Verification items for the finished model (mm, model axes). Face numbers are marked on the shaded views. A direction names the side the tool comes from. Coordinates: 2 decimals unless noted, no trailing zeros. Write each loop counter-clockwise with the first axis right and the second up, starting at its lowest first coordinate (ties: lowest second). Pieces come first, ordered by that corner, then holes. Notation, with made-up numbers: (48.5, -29.75) - (86.5, -29.75) arc R31 ccw to (86.5, -2.75) - close; hole circle Ø10 at (63, 23). An arc over 180 degrees is marked (long way). Use one line per item in the form item = value. Start each with the question number.
(1) Sectioned sample at B-B (x = 46.5). Count the separate pieces of the cut face and the enclosed holes in it, and give its area (3 significant figures).
(2) Material ranges on line 1 (Y direction, x = 51, z = -2.75); line 2 (X direction, y = 10, z = 0.25); line 3 (X direction, y = 15.5, z = -1), recorded low to high. Write a range as [from, to].
(3) Gauge pin test, flat ends, axial feed: pin 1 Ø0.7 at (x, z) = (2, 9.5) entering from +Y; pin 2 Ø4.5 at (y, z) = (12.5, -2.5) entering from -X; pin 3 Ø6 at (x, z) = (40.5, 5) entering from -Y. Record the tip position at first contact, or that the pin passes through.
(4) Tool access check on the marked faces 4, 5 and 6. Record the directions out of +Z, -Z, +X, -X, +Y, -Y that give a thin tool (end or side, any length) a straight path to the whole face; none if there is none.
(5) Mould release check, pull along X, two halves, no side actions. Record for the marked faces 1, 2 and 3: released by +X, released by -X, zero draft, split by the parting line, or undercut.
(6) Sectioned sample at A-A (z = 3.75). Record the cut outline in (x, y), and give its area (3 significant figures).
from build123d import *

# Parameters (mm, degrees)
BOSS_EXTRUDE1_DEPTH  = 10.8
BOSS_EXTRUDE2_DEPTH  = 1
SKETCH3_W            = 2
SKETCH3_H            = 10
BOSS_EXTRUDE3_DEPTH  = 2.3
FILLET1_SIZE         = 2
FILLET1_SIZE_2       = 1
CUT_EXTRUDE1_REACH   = 67.321
SKETCH4_W            = 11.5
SKETCH4_H            = 3
BOSS_EXTRUDE4_DEPTH  = 2.3
CHAMFER1_SIZE        = 1.5
CUT_EXTRUDE2_DEPTH   = 2
BOSS_EXTRUDE6_DEPTH  = 2
FILLET2_R            = 1
BOSS_EXTRUDE36_DEPTH = 1
BOSS_EXTRUDE7_DEPTH  = 1.87
SKETCH11_R           = 2.5
CUT_EXTRUDE3_DEPTH   = 66.681732761


with BuildPart() as part:
    # Sketch1 → Boss-Extrude1 (new body)
    with BuildSketch(Plane.XY):
        with BuildLine():
            ThreePointArc((7.5, 17.5), (2.196699141, 15.303300859), (0, 10))
            Line((0, 10), (0, 0))
            Line((0, 0), (1.5, 0))
            Line((1.5, 0), (1.5, 10))
            ThreePointArc((1.5, 10), (3.257359313, 14.242640687), (7.5, 16))
            Line((7.5, 16), (54.5, 16))
            ThreePointArc((54.5, 16), (58.742640687, 14.242640687), (60.5, 10))
            Line((60.5, 10), (60.5, 0))
            Line((60.5, 0), (62, 0))
            Line((62, 0), (62, 17.5))
            Line((62, 17.5), (7.5, 17.5))
        make_face()
    extrude(amount=BOSS_EXTRUDE1_DEPTH)


with BuildPart() as body_2:
    # Sketch2 → Boss-Extrude2 (new body)
    with BuildSketch(Plane(origin=(0, 0, 0), x_dir=(-1, 0, 0), z_dir=(0, 0, -1))):
        with BuildLine():
            Line((-1.5, 0), (-1.5, 10))
            ThreePointArc((-1.5, 10), (-3.257359313, 14.242640687), (-7.5, 16))
            Line((-7.5, 16), (-54.5, 16))
            ThreePointArc((-54.5, 16), (-58.742640687, 14.242640687), (-60.5, 10))
            Line((-60.5, 10), (-60.5, 0))
            Line((-60.5, 0), (-1.5, 0))
        make_face()
    extrude(amount=-BOSS_EXTRUDE2_DEPTH)

    # Combine1: union part
    add(part.part)

    # Sketch3 → Boss-Extrude3 (add)
    with BuildSketch(Plane.XY.offset(10.8)):
        with Locations((2.5, 5)):
            Rectangle(SKETCH3_W, SKETCH3_H)
        with Locations((59.5, 5)):
            Rectangle(SKETCH3_W, SKETCH3_H)
    extrude(amount=-BOSS_EXTRUDE3_DEPTH)

    # Fillet1
    # a fillet whose section is not a circle: 2, 1 mm, written as the material it takes off along each edge
    with BuildSketch(Plane(origin=(0, 10, 10.8), x_dir=(0, 0, -1), z_dir=(0, -1, 0))) as fillet1_piece_1:
        with BuildLine():
            Bezier((FILLET1_SIZE, 0), (0, 0), (0, FILLET1_SIZE_2), weights=[1, 0.707106781, 1])
            Line((0, FILLET1_SIZE_2), (0, 0))
            Line((0, 0), (FILLET1_SIZE, 0))
        make_face()
    extrude(amount=15, mode=Mode.SUBTRACT)
    with BuildSketch(Plane(origin=(7.5, 10, 10.8), x_dir=(0, 1, 0), z_dir=(1, 0, 0))) as fillet1_piece_2:
        with BuildLine():
            Bezier((7.5, -FILLET1_SIZE), (7.5, 0), (7.5 - FILLET1_SIZE_2, 0), weights=[1, 0.707106781, 1])
            Line((7.5 - FILLET1_SIZE_2, 0), (7.5, 0))
            Line((7.5, 0), (7.5, -FILLET1_SIZE))
        make_face()
    revolve(axis=Axis((7.5, 10, 10.8), (0, 0, 1)), revolution_arc=90, mode=Mode.SUBTRACT)
    with BuildSketch(Plane(origin=(67, 17.5, 10.8), x_dir=(0, 0, -1), z_dir=(-1, 0, 0))) as fillet1_piece_3:
        with BuildLine():
            Bezier((FILLET1_SIZE, 0), (0, 0), (0, FILLET1_SIZE_2), weights=[1, 0.707106781, 1])
            Line((0, FILLET1_SIZE_2), (0, 0))
            Line((0, 0), (FILLET1_SIZE, 0))
        make_face()
    extrude(amount=59.5, mode=Mode.SUBTRACT)

    # Sketch4 → Cut-Extrude1 (cut, up to next)
    with BuildSketch(Plane(origin=(0, 17.5, 0), x_dir=(1, 0, 0), z_dir=(0, 1, 0)), mode=Mode.PRIVATE) as cut_extrude1_sk1:
        with Locations((45.75, -4.55)):
            Rectangle(SKETCH4_W, SKETCH4_H)
    cut_extrude1_tool1 = extrude(cut_extrude1_sk1.sketch, amount=-CUT_EXTRUDE1_REACH, mode=Mode.PRIVATE) & body_2.part
    add(cut_extrude1_tool1.solids().sort_by_distance((45.75, 17.5, 4.55))[0], mode=Mode.SUBTRACT)

    # Sketch5 → Boss-Extrude4 (add)
    with BuildSketch(Plane.XY.offset(10.8)):
        with BuildLine():
            Line((60.5, 10), (59.5, 10))
            ThreePointArc((59.5, 10), (58.035533906, 13.535533906), (54.5, 15))
            Line((54.5, 15), (7.5, 15))
            ThreePointArc((7.5, 15), (3.964466094, 13.535533906), (2.5, 10))
            Line((2.5, 10), (1.5, 10))
            ThreePointArc((1.5, 10), (3.257359313, 14.242640687), (7.5, 16))
            Line((7.5, 16), (54.5, 16))
            ThreePointArc((54.5, 16), (58.742640687, 14.242640687), (60.5, 10))
        make_face()
    extrude(amount=-BOSS_EXTRUDE4_DEPTH)

    # Chamfer1
    chamfer1_edges = [body_2.edges().sort_by_distance(p)[0] for p in [
        (58.035533906, 13.535533906, 10.8),
        (3.964466094, 13.535533906, 10.8),
        (31, 15, 10.8),
    ]]
    chamfer(chamfer1_edges, length=CHAMFER1_SIZE - 0.0001)  # a hair under: the kernel refuses the full size

    # Chamfer3: read off the stored shape, not the designer's step
    # Chamfer3: loft between two sections, ruled curve by curve
    chamfer3_from = [
        Edge.make_three_point_arc((2.4, 10, 9.4), (3.893755416, 13.606244584, 9.4), (7.5, 15.1, 9.4)),
        Edge.make_three_point_arc((54.5, 15.1, 9.4), (58.106244584, 13.606244584, 9.4), (59.6, 10, 9.4)),
        Edge.make_line((7.5, 15.1, 9.4), (54.5, 15.1, 9.4)),
        Edge.make_line((59.6, 10, 9.4), (2.4, 10, 9.4)),
    ]
    chamfer3_to = [
        Edge.make_three_point_arc((1.5, 10, 8.5), (3.257359313, 14.242640687, 8.5), (7.5, 16, 8.5)),
        Edge.make_three_point_arc((54.5, 16, 8.5), (58.742640687, 14.242640687, 8.5), (60.5, 10, 8.5)),
        Edge.make_line((7.5, 16, 8.5), (54.5, 16, 8.5)),
        Edge.make_line((60.5, 10, 8.5), (1.5, 10, 8.5)),
    ]
    chamfer3 = Solid(Shell([*[Face.make_surface_from_curves(chamfer3_from[k], chamfer3_to[k]) for k in range(4)], Face(Wire(chamfer3_from)), Face(Wire(chamfer3_to))]))
    add(chamfer3, mode=Mode.SUBTRACT)

    # Sketch6 → Cut-Extrude2 (cut)
    with BuildSketch(Plane(origin=(0, 0, 0), x_dir=(-1, 0, 0), z_dir=(0, 0, -1))):
        with BuildLine():
            Line((-59.98, 10.15), (-59.98, 16.85))
            Line((-59.98, 16.85), (-59.98, 17.5))
            Line((-59.98, 17.5), (-42.02, 17.5))
            Line((-42.02, 17.5), (-42.02, 16.85))
            Line((-42.02, 16.85), (-42.02, 10.15))
            ThreePointArc((-42.02, 10.15), (-51, 1.17), (-59.98, 10.15))
        make_face()
    extrude(amount=-CUT_EXTRUDE2_DEPTH, mode=Mode.SUBTRACT)

    # Sketch9 → Boss-Extrude6 (add)
    with BuildSketch(Plane(origin=(0, 0, 0), x_dir=(-1, 0, 0), z_dir=(0, 0, -1))):
        with BuildLine():
            Line((-54.5, 0), (-62, 0))
            Line((-62, 0), (-62, 6.85))
            Line((-62, 6.85), (-62, 17.5))
            Line((-62, 17.5), (-59.98, 17.5))
            Line((-59.98, 17.5), (-59.98, 10.15))
            ThreePointArc((-59.98, 10.15), (-51, 1.17), (-42.02, 10.15))
            Line((-42.02, 10.15), (-42.02, 17.5))
            Line((-42.02, 17.5), (-40, 17.5))
            Line((-40, 17.5), (-40, 6.854472052))
            Line((-40, 6.854472052), (-40, 0))
            Line((-40, 0), (-47.292116273, 0))
            Line((-47.292116273, 0), (-54.5, 0))
        make_face()
    extrude(amount=BOSS_EXTRUDE6_DEPTH)

    # Fillet2
    fillet2_edges = [body_2.edges().sort_by_distance(p)[0] for p in [
        (51.5, 17.5, 4.55),
        (45.75, 17.5, 3.05),
        (40, 17.5, 4.55),
        (45.75, 17.5, 6.05),
    ]]
    fillet(fillet2_edges, radius=FILLET2_R)

    # Sketch48 → Boss-Extrude36 (add)
    with BuildSketch(Plane(origin=(0, 0, 2), x_dir=(-1, 0, 0), z_dir=(0, 0, -1))):
        with BuildLine():
            Line((-54.5, 16), (-42.02, 16))
            Line((-42.02, 16), (-42.02, 17.5))
            Line((-42.02, 17.5), (-59.98, 17.5))
            Line((-59.98, 17.5), (-59.98, 12.443276489))
            ThreePointArc((-59.98, 12.443276489), (-57.766522698, 15.032874871), (-54.5, 16))
        make_face()
    extrude(amount=BOSS_EXTRUDE36_DEPTH)

    # Sketch10 → Boss-Extrude7 (add)
    with BuildSketch(Plane(origin=(0, 0, -2), x_dir=(-1, 0, 0), z_dir=(0, 0, -1))):
        Polygon((-54.5, 0), (-62, 0), (-62, 3.4), (-62, 17.5), (-40, 17.5), (-40, 6.854472052), (-40, 0), (-47.292116273, 0), align=None)
    extrude(amount=BOSS_EXTRUDE7_DEPTH)

    # Sketch11 → Cut-Extrude3 (cut, through all)
    with BuildSketch(Plane.XY.offset(-2)):
        with Locations((51, 8.65)):
            Circle(SKETCH11_R)
    extrude(amount=-CUT_EXTRUDE3_DEPTH, mode=Mode.SUBTRACT)


solid = body_2.part
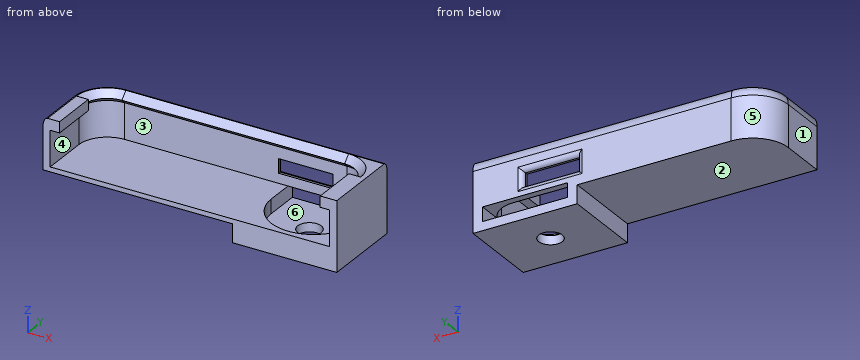
Answers below:
q1.separate_pieces = 3
q1.enclosed_holes = 0
q1.area = 49.9 mm2
q2.line_1 = [0, 6.15], [11.15, 17.5]
q2.line_2 = [0, 42.02], [59.98, 62]
q2.line_3 = [40, 42.02], [59.98, 62]
q3.pin_1 = 15.38
q3.pin_2 = 40
q3.pin_3 = 16
q4.face_4 = -Y
q4.face_5 = +Z, -Z, -X, +Y
q4.face_6 = +Y
q5.face_1 = released by -X
q5.face_2 = zero draft
q5.face_3 = undercut
q6.outline = (0, 0) - (1.5, 0) - (1.5, 10) arc R6 cw to (7.5, 16) - (40, 16) - (40, 16.5) arc R1 ccw to (39, 17.5) - (7.5, 17.5) arc R7.5 ccw to (0, 10) - close; (51.5, 16) - (54.5, 16) arc R6 cw to (60.5, 10) - (60.5, 0) - (62, 0) - (62, 17.5) - (52.5, 17.5) arc R1 ccw to (51.5, 16.5) - close
q6.area = 127 mm2
